The model under review builds one solid part; all positions refer to its coordinate system, in mm. A direction names the side the tool comes from. Round coordinates to 2 decimals unless told otherwise and drop trailing zeros. Loops run counter-clockwise (first coordinate to the right, second up) from the corner with the lowest first, then second, coordinate; pieces in that order, holes last. Notation, with made-up numbers: M 70.25,-38 L 101.25,-38 A24 ccw 101.25,-14 Z; hole C 75,5 d4. An arc over 180 degrees is marked long. Answer as a JSON object with one key per item and string values. Group by question number.
Item 1: The part is to be moulded in two halves that separate along Y. For faces 3 (the face through (37.75, -11.85, -0.09)), 4 (the face through (-82.548, -0.201, -0.089)), 5 (the face through (15.119, 3.155, -0.089)), 6 (the face through (-37.75, 11.85, -0.09)), say which applies: +Y half, -Y half, draft (parallel to the pull), parting line (faces both ways), or undercut.
Item 2: To check wall thickness, follow line 1 (X direction, y = 0, z = -3); line 2 (X direction, y = 0, z = -1); line 3 (Y direction, x = 0, z = -2.5). State the ranges of each line that lie inside material, in increasing order.
Item 3: Consider section D-D (y = 7.25). Give the boundary of the cut face in (x, z), and give its area (3 significant figures).
Item 4: Consider section B-B (x = -12.7). Give the boundary of the cut face in (y, z), and give its area (3 significant figures).
Item 5: Tool access review of faces 1 (the face through (53.976, -0.157, -4.66)), 2 (the face through (-8.82, 0.86, -0.09)): name each direction out of +Z, -Z, +X, -X, +Y, -Y from which nothing blocks a thin tool from reaching the whole face with its end or side.
Item 6: Insertion check: P1, Ø5, axis at y = -7, z = 3, coming from the -X side; P2, Ø6.5, axis at x = 65, y = 1, coming from the -Z side. Each pin has a flat end and moves straight along its axis. Give the tip position at first contact, or say it passes through.
Item 7: Consider section C-C (z = -1.5). State how many separate pieces and enclosed holes the cut face has, and give its area (3 significant figures).
Item 8: Consider section A-A (y = 0). Give the boundary of the cut face in (x, z).
Autodesk Inventor part; units mm, degrees
ref_plane "YZ Plane" through (0, 0, 0) normal (1, 0, 0) x (0, 1, 0)
ref_plane "XZ Plane" through (0, 0, 0) normal (0, 1, 0) x (-1, 0, 0)
ref_plane "XY Plane" through (0, 0, 0) normal (0, 0, 1) x (1, 0, 0)
sketch "Sketch2" plane through (0, 0, 0) normal (0, 0, 1) x (1, 0, 0)
  line L0 (-73.6458, 9.5048) -> (-0.8277, 14.2605)
  arc A0 (0.8277, 14.2605) -> (-0.8277, 14.2605) centre (0, 1.5875) ccw
  line L1 (0.8277, 14.2605) -> (73.6458, 9.5048)
  arc A1 (73.6458, -9.5048) -> (73.6458, 9.5048) centre (73.025, 0) ccw
  line L2 (73.6458, -9.5048) -> (0.8277, -14.2605)
  arc A2 (-0.8277, -14.2605) -> (0.8277, -14.2605) centre (0, -1.5875) ccw
  line L3 (-0.8277, -14.2605) -> (-73.6458, -9.5048)
  arc A3 (-73.6458, 9.5048) -> (-73.6458, -9.5048) centre (-73.025, 0) ccw
  line L4 (-73.025, 0) -> (73.025, 0) construction
  line L5 (0, 20.0025) -> (0, -20.0025) construction
  line L6 (0, 1.5875) -> (0, -1.5875) construction
  point P0 (0, 0)
  point P1 (0, 0)
  dimension "d0" = 3.175
  dimension "d1" = 12.7
  dimension "d2" = 9.525
  dimension "d3" = 146.05
extrude "Extrusion1" add sketch "Sketch2" along normal mid plane 12.7
sketch "Sketch3" plane through (0, 0, 6.35) normal (0, 0, 1) x (1, 0, 0)
  line L0 (-12.7, 0) -> (12.7, 0) construction
  point P0 (0, 0)
  point P1 (0, 0)
  point P2 (0, 0)
  dimension "d6" = 25.4
hole "Hole1" at (0, 0, 6.35) at (-12.7, 0, 6.35) at (12.7, 0, 6.35) direction (0, 0, -1) diameter 7.9502 end through all
sketch "Sketch7" plane through (0, 0, 6.35) normal (0, 0, 1) x (1, 0, 0)
  arc A0 (-73.6458, 9.5048) -> (-73.6458, -9.5048) centre (-73.025, 0) ccw construction
  point P0 (0, 0)
hole "Hole4" at (-73.025, 0, 6.35) direction (0, 0, -1) diameter 9.525 end through all
sketch "Sketch9" plane through (0, 0, -6.35) normal (0, 0, -1) x (-1, 0, 0)
  circle A0 centre (73.025, 0) radius 4.7625 construction
  circle A1 centre (-12.7, 0) radius 3.9751 construction
  circle A2 centre (12.7, 0) radius 3.9751 construction
  circle A3 centre (0, 0) radius 3.9751 construction
  line L0 (-73.6458, -9.5048) -> (-0.8277, -14.2605)
  arc A4 (-0.8277, -14.2605) -> (0.8277, -14.2605) centre (0, -1.5875) ccw construction
  line L1 (0.8277, -14.2605) -> (73.6458, -9.5048) construction
  arc A5 (73.6458, -9.5048) -> (73.6458, 9.5048) centre (73.025, 0) ccw construction
  line L2 (73.6458, 9.5048) -> (0.8277, 14.2605) construction
  arc A6 (0.8277, 14.2605) -> (-0.8277, 14.2605) centre (0, 1.5875) ccw construction
  line L3 (-0.8277, 14.2605) -> (-73.6458, 9.5048)
  arc A7 (-73.6458, 9.5048) -> (-73.6458, -9.5048) centre (-73.025, 0) ccw
  arc A8 (-57.183, -10.5799) -> (-57.183, 10.5799) centre (-73.025, 0) ccw
  dimension "d48" = 19.05
extrude "Extrusion3" cut sketch "Sketch9" against normal blind 3.429
sketch "Sketch8" plane through (0, 0, 6.35) normal (0, 0, 1) x (1, 0, 0)
  arc A0 (73.6458, -9.5048) -> (73.6458, 9.5048) centre (73.025, 0) ccw construction
  point P0 (0, 0)
  point P1 (73.025, 0)
hole "Hole5" at (73.025, 0, 6.35) direction (0, 0, -1) diameter 6.35 end through all
equation "\"d46\" = d0"
properties part number "PLATE,ROCKER,ELEVATOR" material "Aluminum, 7075-T6"
Geometry results:
{
 "1": {"face 3": "-Y half", "face 4": "parting line", "face 5": "undercut", "face 6": "+Y half"},
 "2": {"line 1": "x = -82.55 to -77.79, -68.26 to -16.68, -8.72 to -3.98, 3.98 to 8.72, 16.68 to 53.97", "line 2": "x = -82.55 to -77.79, -68.26 to -16.68, -8.72 to -3.98, 3.98 to 8.72, 16.68 to 69.85, 76.2 to 82.55", "line 3": "y = -14.29 to -3.98, 3.98 to 14.29"},
 "3": {"outline": "M -79.2,-6.35 L 55.41,-6.35 L 55.41,-2.92 L 79.2,-2.92 L 79.2,6.35 L -79.2,6.35 Z", "area": "1,930 mm^2"},
 "4": {"outline": "M -13.49,-6.35 L -3.98,-6.35 L -3.98,6.35 L -13.49,6.35 Z; M 3.98,-6.35 L 13.49,-6.35 L 13.49,6.35 L 3.98,6.35 Z", "area": "242 mm^2"},
 "5": {"face 1": "-Z, +X", "face 2": "+Z, -Z"},
 "6": {"P1": "stops at x = -81.42", "P2": "stops at z = -2.92"},
 "7": {"separate pieces": "1", "enclosed holes": "5", "area": "3,520 mm^2"},
 "8": {"outline": "M -82.55,-6.35 L -77.79,-6.35 L -77.79,6.35 L -82.55,6.35 Z; M -68.26,-6.35 L -16.68,-6.35 L -16.68,6.35 L -68.26,6.35 Z; M -8.72,-6.35 L -3.98,-6.35 L -3.98,6.35 L -8.72,6.35 Z; M 3.98,-6.35 L 8.72,-6.35 L 8.72,6.35 L 3.98,6.35 Z; M 16.68,-6.35 L 53.97,-6.35 L 53.97,-2.92 L 69.85,-2.92 L 69.85,6.35 L 16.68,6.35 Z; M 76.2,-2.92 L 82.55,-2.92 L 82.55,6.35 L 76.2,6.35 Z"}
}
